```python
from build123d import *

# Parameters (mm, degrees)
SKETCH1_W                  = 135
SKETCH1_H                  = 210
BOSS_EXTRUDE1_DEPTH        = 10
CUT_EXTRUDE1_START         = -8
SKETCH4_W                  = 135
SKETCH4_H                  = 10
CUT_EXTRUDE1_DEPTH         = 3
SKETCH15_W                 = 35
SKETCH15_H                 = 160
CUT_EXTRUDE2_DEPTH         = 11
SKETCH16_R                 = 1.5
CUT_EXTRUDE3_DEPTH         = 5
CUT_EXTRUDE4_DEPTH         = 5.4
F_3_0_3_DIAMETER_HOLE1_D   = 3
LPATTERN4_COUNT            = 2
LPATTERN4_PITCH            = 16
LPATTERN4_COUNT_DIR2       = 3
LPATTERN4_PITCH_DIR2       = 25
LPATTERN1_COUNT            = 3
LPATTERN1_PITCH            = 50
F_5_5_5_5_DIAMETER_HOLE1_D = 5.5
LPATTERN3_COUNT            = 3
LPATTERN3_PITCH            = 50
FILLET1_R                  = 15


with BuildPart() as part:
    # Sketch1 → Boss-Extrude1 (new body)
    with BuildSketch(Plane(origin=(0, 0, 0), x_dir=(0, 0, -1), z_dir=(1, 0, 0))):
        with Locations((67.5, 105)):
            Rectangle(SKETCH1_W, SKETCH1_H)
    extrude(amount=BOSS_EXTRUDE1_DEPTH)

    # Sketch4 → Cut-Extrude1 (cut, through all)
    with BuildSketch(Plane(origin=(10, 0, 0), x_dir=(0, 0, -1), z_dir=(1, 0, 0)).offset(CUT_EXTRUDE1_START)):
        with Locations((67.5, 5)):
            Rectangle(SKETCH4_W, SKETCH4_H)
        with Locations((67.5, 205)):
            Rectangle(SKETCH4_W, SKETCH4_H)
    extrude(amount=-CUT_EXTRUDE1_DEPTH, mode=Mode.SUBTRACT)

    # Sketch15 → Cut-Extrude2 (cut, through all)
    with BuildSketch(Plane(origin=(10, 0, 0), x_dir=(0, 0, -1), z_dir=(1, 0, 0))):
        with Locations((32.5, 105)):
            Rectangle(SKETCH15_W, SKETCH15_H)
        with Locations((102.5, 105)):
            Rectangle(SKETCH15_W, SKETCH15_H)
    extrude(amount=-CUT_EXTRUDE2_DEPTH, mode=Mode.SUBTRACT)

    # Sketch16 → Cut-Extrude3 (cut)
    with BuildSketch(Plane(origin=(10, 0, 0), x_dir=(0, 0, -1), z_dir=(1, 0, 0))):
        with Locations((67.5, 100)):
            Circle(SKETCH16_R)
        with Locations((67.5, 150)):
            Circle(SKETCH16_R)
    extrude(amount=-CUT_EXTRUDE3_DEPTH, mode=Mode.SUBTRACT)

    # Sketch6 → Cut-Extrude4 (cut)
    with BuildSketch(Plane.ZY.offset(-10)):
        with BuildLine():
            Line((-22.25, 5), (-22.25, 0))
            Line((-22.25, 0), (-12.75, 0))
            Line((-12.75, 0), (-12.75, 5))
            ThreePointArc((-12.75, 5), (-17.5, 9.75), (-22.25, 5))
        make_face()
        with BuildLine():
            Line((-22.25, 205), (-22.25, 210))
            Line((-22.25, 210), (-12.75, 210))
            Line((-12.75, 210), (-12.75, 205))
            ThreePointArc((-12.75, 205), (-17.5, 200.25), (-22.25, 205))
        make_face()
    cut_extrude4 = extrude(amount=CUT_EXTRUDE4_DEPTH, mode=Mode.SUBTRACT)

    # Ø3.0 (3) Diameter Hole1 (through all)
    with Locations(Plane(origin=(10, 0, 0), x_dir=(0, 0, -1), z_dir=(1, 0, 0))):
        with Locations((59.5, 100)):
            f_3_0_3_diameter_hole1 = Hole(F_3_0_3_DIAMETER_HOLE1_D / 2)

    # LPattern4: 3.0 _3_ Diameter Hole1 2 × 3
    with Locations(*[(0, j * LPATTERN4_PITCH_DIR2, -i * LPATTERN4_PITCH) for i in range(LPATTERN4_COUNT) for j in range(LPATTERN4_COUNT_DIR2) if (i, j) != (0, 0)]):
        add(f_3_0_3_diameter_hole1, mode=Mode.SUBTRACT)

    # LPattern1: Cut-Extrude4 ×3
    with Locations(*[(0, 0, -i * LPATTERN1_PITCH) for i in range(1, LPATTERN1_COUNT)]):
        add(cut_extrude4, mode=Mode.SUBTRACT)

    # Ø5.5 (5.5) Diameter Hole1 (through all)
    with Locations(Plane(origin=(4.6, 0, 0), x_dir=(0, 0, -1), z_dir=(1, 0, 0))):
        with Locations((17.5, 205), (17.5, 5)):
            f_5_5_5_5_diameter_hole1 = Hole(F_5_5_5_5_DIAMETER_HOLE1_D / 2)

    # LPattern3: Ø5.5 (5.5) Diameter Hole1 ×3
    with Locations(*[(0, 0, -i * LPATTERN3_PITCH) for i in range(1, LPATTERN3_COUNT)]):
        add(f_5_5_5_5_diameter_hole1, mode=Mode.SUBTRACT)

    # Fillet1
    fillet1_edges = [part.edges().sort_by_distance(p)[0] for p in [
        (5, 25, -15),
        (5, 185, -15),
        (5, 185, -50),
        (5, 25, -50),
        (5, 25, -85),
        (5, 185, -85),
        (5, 185, -120),
        (5, 25, -120),
    ]]
    fillet(fillet1_edges, radius=FILLET1_R)


solid = part.part
```
Build history of the part. All positions in model axes, mm. A direction names the side the tool comes from. Give positions to 0.01 mm unless a question says otherwise; leave off trailing zeros.
Item 1: Flat gauge pins, fed straight in: pin 1 (5 mm diameter, centred on y = 4.5, z = -117, fed in from +X); pin 2 (2.5 mm diameter, centred on y = 150, z = -67.5, fed in from +X); pin 3 (0.6 mm diameter, centred on x = 0.5, z = -78.5, fed in from +Y). Where does each tip first touch, or does it go through?
Answers follow:
pin 1: stops at x = 4.6
pin 2: stops at x = 5
pin 3: stops at y = 200
Item 2: Drill centre lines: line 1 (Y direction, x = 3.75, z = -75.5); line 2 (Z direction, x = 4.25, y = 150); line 3 (Y direction, x = 7.1, z = -67.5). Where is each one in solid material? Low to high.
Answers follow:
line 1: y = 0 to 98.5, 101.5 to 123.5, 126.5 to 148.5, 151.5 to 210
line 2: z = -135 to -120, -85 to -77, -74 to -61, -58 to -50, -15 to 0
line 3: y = 9.75 to 98.5, 101.5 to 148.5, 151.5 to 200.25
Item 3: Slice it at A-A, the plane x = 7.25. Give the number of separate pieces and of enclosed holes in the cut face, and give its area (3 significant figures).
Answers follow:
separate pieces: 1
enclosed holes: 10
area: 17,000 mm2
Item 4: Pull direction Y, two halves, no side cores. Call faces 5 (the face through (7.34, 9.75, -117.4)), 6 (the face through (3.282, 202.315, -18.096)), 7 (the face through (7, 208, -62.75)), 8 (the face through (3.282, 5.121, -70.247)): released by +Y, released by -Y, zero draft, split by the parting line, or undercut.
Answers follow:
face 5: released by -Y
face 6: undercut
face 7: zero draft
face 8: undercut
Item 5: Which spindle directions (+Z, -Z, +X, -X, +Y, -Y) get a long thin tool onto all of the face, cutting with end or side? Do faces 1 (the face through (4.6, 3, -15)), 2 (the face through (5, 104, -120)), 3 (the face through (7, 208, -112.75)), 4 (the face through (2, 8, -67)). Say none if no direction does.
Answers follow:
face 1: +X, -Y
face 2: +X, -X
face 3: +X, +Y
face 4: +Z, -Z, -X, -Y
